Input: part model. Units: mm. Frame: model coordinates. Face numbers are marked on the shaded views. A direction names the side the tool comes from. Give positions to 0.01 mm unless a question says otherwise; leave off trailing zeros. Loops run counter-clockwise (first coordinate to the right, second up) from the corner with the lowest first, then second, coordinate; pieces in that order, holes last.
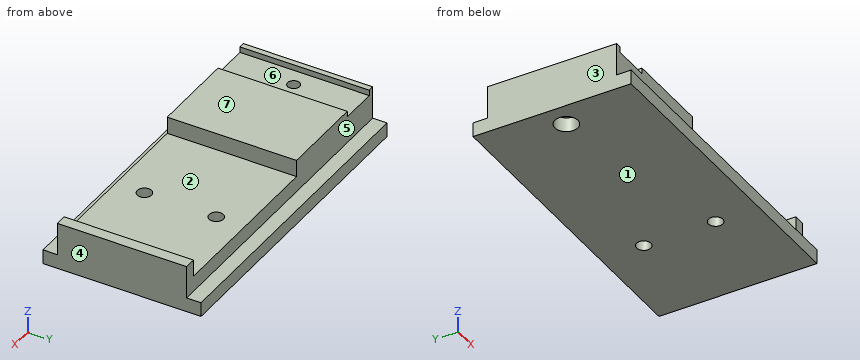
from build123d import *

# Parameters (mm, degrees)
F0_W           = 110
F0_H           = 55
F1_DEPTH       = 5
F2_W           = 110
F2_H           = 45
F3_DEPTH       = 11.4
F4_W           = 13
F4_H           = 45
F5_DEPTH       = 2
F4_W_2         = 61
F6_DEPTH       = 5.9
F8_D           = 4.2
F8_CBORE_D     = 8
F8_CBORE_DEPTH = 5
F10_D          = 5


with BuildPart() as f1:
    # F0 (on Top) → F1 (new body)
    with BuildSketch(Plane.XY):
        Rectangle(F0_W, F0_H)
    extrude(amount=F1_DEPTH)

    # F2 (on face) → F3 (join)
    with BuildSketch(Plane.XY.offset(5)):
        Rectangle(F2_W, F2_H)
    extrude(amount=F3_DEPTH)

    # F4 (on face) → F5 (cut)
    with BuildSketch(Plane.XY.offset(16.4)):
        with Locations((-46.5, 0)):
            Rectangle(F4_W, F4_H)
    extrude(amount=-F5_DEPTH, mode=Mode.SUBTRACT)

    # F4 (on face) → F6 (cut)
    with BuildSketch(Plane.XY.offset(16.4)):
        with Locations((20.5, 0)):
            Rectangle(F4_W_2, F4_H)
    extrude(amount=-F6_DEPTH, mode=Mode.SUBTRACT)

    # F8 (through all)
    with Locations(Plane(origin=(0, 0, 0), x_dir=(1, 0, 0), z_dir=(0, 0, -1))):
        with Locations((-46.5, 0)):
            CounterBoreHole(F8_D / 2, F8_CBORE_D / 2, F8_CBORE_DEPTH)

    # F10 (through all)
    with Locations(Plane.XY.offset(10.5)):
        with Locations((20.5, 12.5), (20.5, -12.5)):
            Hole(F10_D / 2)


solid = f1.part
(1) Cut plane C-C (x = 20.5). Return the cut outline in (y, z).
Values follow:
outline: (-27.5, 0) - (-15, 0) - (-15, 10.5) - (-22.5, 10.5) - (-22.5, 5) - (-27.5, 5) - close; (-10, 0) - (10, 0) - (10, 10.5) - (-10, 10.5) - close; (15, 0) - (27.5, 0) - (27.5, 5) - (22.5, 5) - (22.5, 10.5) - (15, 10.5) - close
(2) Cut plane A-A (z = 13). Return the cut outline in (x, y).
Values follow:
outline: (-55, -22.5) - (-10, -22.5) - (-10, 22.5) - (-55, 22.5) - close; (51, -22.5) - (55, -22.5) - (55, 22.5) - (51, 22.5) - close; hole circle Ø4.2 at (-46.5, 0)
(3) Pin query (flat end, axial travel): pin 1 Ø4 at (x, y) = (25.5, -11) entering from +Z; pin 2 Ø2.5 at (x, y) = (-44.5, 1) entering from -Z; pin 3 Ø4 at (x, y) = (-48, -1.5) entering from +Z. Return the tip coordinate at first contact, or that it passes through.
Values follow:
pin 1: stops at z = 10.5
pin 2: stops at z = 5
pin 3: stops at z = 14.4
(4) Mould query, pull axis X, two halves, no side actions, for the marked faces 1, 2, 3 and 4. Classes: +X half, -X half, draft (parallel to the pull), parting line (faces both ways), or undercut.
Values follow:
face 1: draft
face 2: undercut
face 3: -X half
face 4: +X half
(5) Cut plane D-D (x = -46.5). Return the cut outline in (y, z), and give its area (3 significant figures).
Values follow:
outline: (-27.5, 0) - (-4, 0) - (-4, 5) - (-2.1, 5) - (-2.1, 14.4) - (-22.5, 14.4) - (-22.5, 5) - (-27.5, 5) - close; (2.1, 5) - (4, 5) - (4, 0) - (27.5, 0) - (27.5, 5) - (22.5, 5) - (22.5, 14.4) - (2.1, 14.4) - close
area: 619 mm2
(6) Reachability of the marked faces 5, 6 and 7 from +Z, -Z, +X, -X, +Y, -Y: full face, straight path, thin tool, end or side. Return the list, or none.
Values follow:
face 5: +Z, +X, -X, +Y
face 6: +Z, +Y, -Y
face 7: +Z, +X, -X, +Y, -Y
(7) Ray query, probe 1 along X at (y, z) = (11, 14.75); probe 2 along Y at (x, z) = (-46.5, 7.5); probe 3 along X at (y, z) = (-2.5, 12.75). Return the intervals inside material, ascending.
Values follow:
probe 1: x = -55 to -53, -40 to -10, 51 to 55
probe 2: y = -22.5 to -2.1, 2.1 to 22.5
probe 3: x = -55 to -10, 51 to 55
(8) Cut plane B-B (y = 0). Return the cut outline in (x, z).
Values follow:
outline: (-55, 0) - (-50.5, 0) - (-50.5, 5) - (-48.6, 5) - (-48.6, 14.4) - (-53, 14.4) - (-53, 16.4) - (-55, 16.4) - close; (-44.4, 5) - (-42.5, 5) - (-42.5, 0) - (55, 0) - (55, 16.4) - (51, 16.4) - (51, 10.5) - (-10, 10.5) - (-10, 16.4) - (-40, 16.4) - (-40, 14.4) - (-44.4, 14.4) - close
